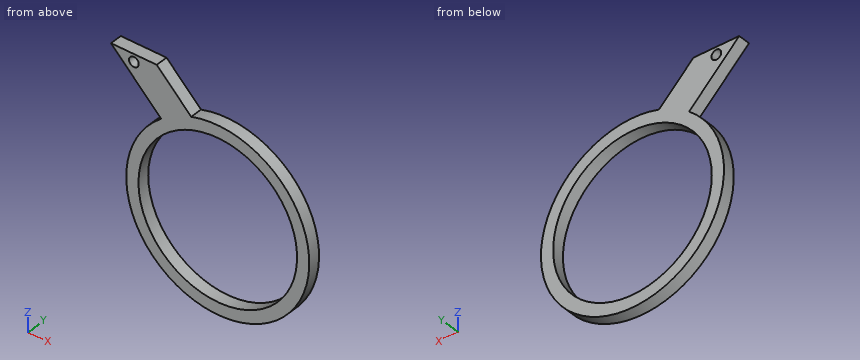
Autodesk Inventor part; units mm, degrees
ref_plane "YZ Plane" through (0, 0, 0) normal (1, 0, 0) x (0, 1, 0)
ref_plane "XZ Plane" through (0, 0, 0) normal (0, 1, 0) x (-1, 0, 0)
ref_plane "XY Plane" through (0, 0, 0) normal (0, 0, 1) x (1, 0, 0)
sketch "Sketch1" plane through (0, 0, 0) normal (0, 1, 0) x (-1, 0, 0)
  line L0 (0, 0) -> (15, 0)
  circle A0 centre (7.5, -2.5) radius 1.6
  line L1 (15, 0) -> (44.3967, 0) construction
  line L2 (0, 0) -> (21.2132, 0) construction
  circle A1 centre (-20, -40) radius 26
  arc A2 (-11.2917, -11.2917) -> (-1.4346, -16.4346) centre (-20, -40) ccw
  line L3 (15, 0) -> (-1.4346, -16.4346)
  line L4 (0, 0) -> (-11.2917, -11.2917)
  line L5 (0, 0) -> (15.9689, 0) construction
  dimension "d0" = 15
  dimension "d1" = 2.5
  dimension "d2" = 7.5
  dimension "d3" = 3.2
  dimension "d6" = 52
  dimension "d7" = 40
  dimension "d8" = 60
  dimension "d10" = 20
  dimension "d11" = 135
extrude "Extrusion1" add sketch "Sketch1" along normal blind 4
sketch "Sketch2" plane through (0, 4, 0) normal (0, 1, 0) x (1, 0, 0)
  point P0 (0, 0)
properties part number "Float Walls"
Input: part model. Units: mm. Frame: model coordinates. Round coordinates to 2 decimals unless told otherwise and drop trailing zeros. Order: outer loops, then holes, each group sorted by start corner. A loop starts at its lowest first (then second) coordinate and runs counter-clockwise, first axis right, second up. Notation, with made-up numbers: (67.5, 58.25) - (74.5, 58.25) arc R14 cw to (74.5, 77.25) - close; hole circle Ø10 at (-12, 75). An arc over 180 degrees is marked (long way). Answer as a JSON object with one key per item and string values. Group by question number.
(1) Cut plane B-B (z = -42). Return loops of the section in (x, y), then the cut area to 3 significant figures.
(2) Cut plane D-D (y = 2.75). Return loops of the section in (x, z).
(3) Material intervals for probe 1 along Z at (x, y) = (-4, 0.35); probe 2 along Z at (x, y) = (-7.5, 1.8); probe 3 along Z at (x, y) = (20, 2.05), sorted ascending. Write a range as from..to.
(4) Cut plane C-C (x = -7.5). Return loops of the section in (y, z), then the cut area to 3 significant figures.
(5) Pin query (flat end, axial travel): P1, Ø8, axis at x = 42.5, z = -14, coming from the -Y side; P2, Ø1, axis at y = 0.5, z = -8, coming from the -X side; P3, Ø1.5, axis at y = 3, z = -32.5, coming from the -X side. Return the tip coordinate at first contact, or that it passes through.
(6) Cut plane A-A (x = 20). Return loops of the section in (y, z), then the cut area to 3 significant figures.
Here are the results:
{
 "1": {"outline": "(-9.93, 0) - (-5.92, 0) - (-5.92, 4) - (-9.93, 4) - close; (45.92, 0) - (49.93, 0) - (49.93, 4) - (45.92, 4) - close", "area": "32.1 mm^2"},
 "2": {"outline": "(-15, 0) - (1.43, -16.43) arc R30 ccw (long way) to (11.29, -11.29) - (0, 0) - close; hole circle Ø3.2 at (-7.5, -2.5); hole circle Ø52 at (20, -40)"},
 "3": {"probe 1": "z = -58..-50, -30..-22, -11..0", "probe 2": "z = -51.99..-28.01, -7.5..-4.1, -0.9..0", "probe 3": "z = -70..-66, -14..-10"},
 "4": {"outline": "(0, -51.99) - (4, -51.99) - (4, -28.01) - (0, -28.01) - close; (0, -7.5) - (4, -7.5) - (4, -4.1) - (0, -4.1) - close; (0, -0.9) - (4, -0.9) - (4, 0) - (0, 0) - close", "area": "113 mm^2"},
 "5": {"P1": "passes through", "P2": "stops at x = -7.5", "P3": "stops at x = -9.23"},
 "6": {"outline": "(0, -70) - (4, -70) - (4, -66) - (0, -66) - close; (0, -14) - (4, -14) - (4, -10) - (0, -10) - close", "area": "32.0 mm^2"}
}
